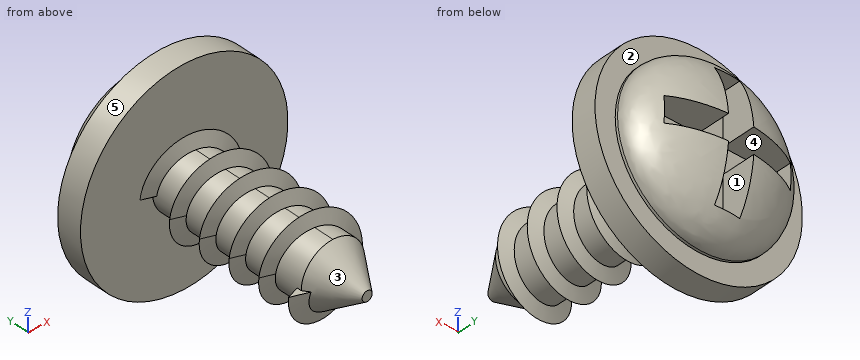
from build123d import *

# Parameters (mm, degrees)
SKETCH1_R           = 4.1
BOSS_EXTRUDE1_DEPTH = 1
SKETCH2_R           = 3.3
BOSS_EXTRUDE2_DEPTH = 0.1
DOME1_FACE_RADIUS   = 3.3
DOME1_HEIGHT        = 1.8
CUT_EXTRUDE1_DEPTH  = 3.5
SKETCH4_R           = 1.25
BOSS_EXTRUDE3_DEPTH = 8
CHAMFER1_SIZE       = 1.5
CHAMFER1_SIZE2      = 1.050311307
SWEEP1_PITCH        = 1.3


with BuildPart() as part:
    # Sketch1 → Boss-Extrude1 (new body)
    with BuildSketch(Plane(origin=(0, 0, 0), x_dir=(1, 0, 0), z_dir=(0, 1, 0))):
        with Locations(Location((0, 0, 0), (0, 0, 270))):
            Circle(SKETCH1_R)
    extrude(amount=BOSS_EXTRUDE1_DEPTH)

    # Sketch2 → Boss-Extrude2 (add)
    with BuildSketch(Plane(origin=(0, 1, 0), x_dir=(1, 0, 0), z_dir=(0, 1, 0))):
        with Locations(Location((0, 0, 0), (0, 0, 270))):
            Circle(SKETCH2_R)
    extrude(amount=BOSS_EXTRUDE2_DEPTH)

    # Dome1: an elliptical dome of height H over a round flat face of radius A is half a spheroid: the quarter ellipse of half axes A and H revolved about the face's axis
    with BuildSketch(Plane((0, 1.1, 0), x_dir=(0, 0, -1), z_dir=(1, 0, 0)), mode=Mode.PRIVATE) as dome1_quarter:
        Ellipse(DOME1_FACE_RADIUS, DOME1_HEIGHT)
        Rectangle(DOME1_FACE_RADIUS, DOME1_HEIGHT, align=(Align.MIN, Align.MIN), mode=Mode.INTERSECT)
    revolve(dome1_quarter.sketch, axis=Axis((0, 1.1, 0), (0, 1, 0)))

    # Sketch3 → Cut-Extrude1 (cut)
    with BuildSketch(Plane(origin=(0, 5, 0), x_dir=(-1, 0, 0), z_dir=(0, 1, 0))):
        Polygon((-0.5, 2.5), (0.5, 2.5), (0.5, 0.5), (2.5, 0.5), (2.5, -0.5), (0.5, -0.5), (0.5, -2.5), (-0.5, -2.5), (-0.5, -0.5), (-2.5, -0.5), (-2.5, 0.5), (-0.5, 0.5), align=None)
    extrude(amount=-CUT_EXTRUDE1_DEPTH, mode=Mode.SUBTRACT)

    # Sketch4 → Boss-Extrude3 (add)
    with BuildSketch(Plane.XZ):
        with Locations(Location((0, 0, 0), (0, 0, 90))):
            Circle(SKETCH4_R)
    extrude(amount=BOSS_EXTRUDE3_DEPTH)

    # Chamfer1
    chamfer1_edges = [part.edges().sort_by_distance(p)[0] for p in [
        (0, -8, -1.25),
    ]]
    chamfer1_side = [part.faces().sort_by_distance(p)[0] for p in [
        (0, -4, -1.25),
    ]]
    chamfer(chamfer1_edges, length=CHAMFER1_SIZE, length2=CHAMFER1_SIZE2, reference=chamfer1_side[0])

    # Sweep1: the profile of Sketch6 screwed along a left-hand helix of 5 turns, 8 arcs to a turn; built about Z, then put on its axis
    sweep1_z = Axis((0, 0, 0), (0, 0, 1))
    sweep1_corners = [(1.75, 0, 0), (1.047756447, 0, -0.25559575), (1.047756447, 0, 0.25559575)]
    with BuildLine(mode=Mode.PRIVATE) as sweep1_profile:
        Line(sweep1_corners[0], sweep1_corners[1])
        Line(sweep1_corners[1], sweep1_corners[2])
        Line(sweep1_corners[2], sweep1_corners[0])
    sweep1_cap = Face(sweep1_profile.wire())
    sweep1_turn_angles = [0, -22.5, -45, -67.5, -90, -112.5, -135, -157.5, -180, -202.5, -225, -247.5, -270, -292.5, -315, -337.5, -360]
    sweep1_turn_weights = [1, 0.9238795325112867, 1, 0.9238795325112867, 1, 0.9238795325112867, 1, 0.9238795325112867, 1, 0.9238795325112867, 1, 0.9238795325112867, 1, 0.9238795325112867, 1, 0.9238795325112867, 1]
    sweep1_turn_rails = [Edge.make_bspline([Vector(p[0], p[1], 0).rotate(sweep1_z, sweep1_turn_angles[k]) / sweep1_turn_weights[k] + Vector(0, 0, p[2] + -SWEEP1_PITCH * sweep1_turn_angles[k] / 360) for k in range(17)], [0, 0, 0, 1, 1, 2, 2, 3, 3, 4, 4, 5, 5, 6, 6, 7, 7, 8, 8, 8], 2, sweep1_turn_weights) for p in sweep1_corners]
    sweep1_turn_sides = [Face.make_surface_from_curves(sweep1_turn_rails[p[0]], sweep1_turn_rails[p[1]]) for p in [(0, 1), (1, 2), (2, 0)]]
    sweep1 = Plane(origin=(0, 0, 0), x_dir=(-1, 0, 0), z_dir=(0, -1, 0)) * Solid(Shell([*[p.moved(Location((0, 0, SWEEP1_PITCH * i))) for i in range(5) for p in sweep1_turn_sides], sweep1_cap, sweep1_cap.rotate(sweep1_z, -1800).moved(Location((0, 0, -SWEEP1_PITCH * -1800 / 360)))]))
    add(sweep1)


solid = part.part
Verification items for the finished model (mm, model axes). Face numbers are marked on the shaded views. A direction names the side the tool comes from. Round coordinates to 2 decimals unless told otherwise and drop trailing zeros. Order: outer loops, then holes, each group sorted by start corner. A loop starts at its lowest first (then second) coordinate and runs counter-clockwise, first axis right, second up.
1. Release check for a two-part mould opening along Z. For the marked faces 1, 2 and 3 record: +Z half, -Z half, draft (parallel to the pull), parting line (faces both ways), or undercut.
Final values:
face 1: undercut
face 2: draft
face 3: parting line
2. Access from +Z, -Z, +X, -X, +Y, -Y to the whole of each face (thin tool, end or side, straight path). Record for the marked faces 4 and 5.
Final values:
face 4: +Y
face 5: +Y, -Y
3. Section check C-C on x = -3.5. Record the cut outline in (y, z).
Final values:
outline: (0, -2.14) - (1, -2.14) - (1, 2.14) - (0, 2.14) - close
4. Go/stop test with flat-tipped pins: P1, Ø0.9, axis at y = 2, z = 0, coming from the +X side; P2, Ø4, axis at y = -6, z = 2, coming from the -X side; P3, Ø1.5, axis at x = 3, z = -2.5, coming from the +Y side. Record where each tip stops, or that it passes through.
Final values:
P1: stops at x = 3.2
P2: stops at x = -1.74
P3: stops at y = 1.63
5. Section check A-A on z = -1.5. State how many separate pieces and enclosed holes the cut face has, then the cut area to 3 significant figures.
Final values:
separate pieces: 6
enclosed holes: 0
area: 15.5 mm2
6. Thickness scan on L1, parallel to Y at x = 0.25, z = 3.75; L2, parallel to X at y = -5.5, z = 0.5; L3, parallel to X at y = 1.25, z = -2.25. Record the ranges inside material, lowest first.
Final values:
L1: y = 0 to 1
L2: x = -1.15 to 1.15
L3: x = -2.4 to 2.4
